```python
from build123d import *

# Parameters (mm, degrees)
F0_W           = 90
F0_H           = 25
F1_DEPTH       = 40
F3_D           = 8.8
F3_CBORE_D     = 14.25
F3_CBORE_DEPTH = 20
F4_T1_DEPTH    = 115.7168298797
F6_D           = 6.8


# Not quite as in the source:
# - a fillet or chamfer that OpenCascade refuses, or shapes differently, is made with other operations: its cross-section is extruded or revolved along the edge and cut away or added


with BuildPart() as f1:
    # F0 (on Front) → F1 (new body)
    with BuildSketch(Plane.XZ):
        with Locations((45, 12.5)):
            Rectangle(F0_W, F0_H)
    extrude(amount=F1_DEPTH)

    # F3 (through all)
    with Locations(Plane.XZ.offset(40)):
        with Locations((22.5, 15), (67.5, 15)):
            CounterBoreHole(F3_D / 2, F3_CBORE_D / 2, F3_CBORE_DEPTH)

    # F4: chamfer of 5 on 1 edges, made by hand

    # F4_s2 → F4_t1 (cut)
    with BuildSketch(Plane.YZ.offset(-12.8584149398)):
        Polygon((-35, 25), (-40, 20), (-40, 25), align=None)
    extrude(amount=F4_T1_DEPTH, mode=Mode.SUBTRACT)

    # F6 (through all)
    with Locations(Plane.XY.offset(25)):
        with Locations((15.8117040992, -15.4151152819), (68.1231990457, -15.4151152819)):
            Hole(F6_D / 2)


solid = f1.part
```
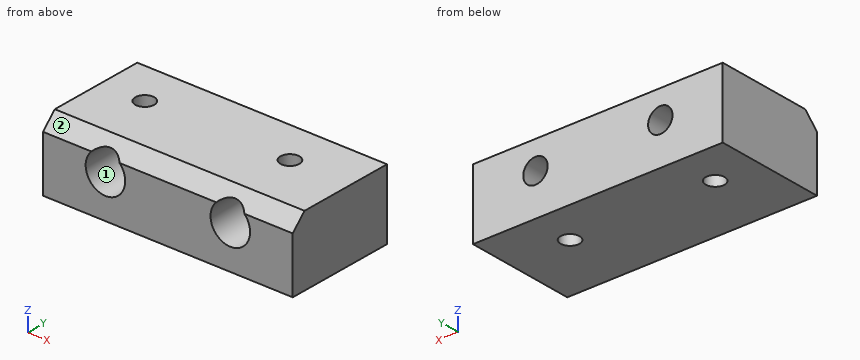
Check sheet for the modelled part. Datum: model origin and axes. Units: mm. Face numbers are marked on the shaded views. A direction names the side the tool comes from. Round coordinates to 2 decimals unless told otherwise and drop trailing zeros. Write each loop counter-clockwise with the first axis right and the second up, starting at its lowest first coordinate (ties: lowest second). Pieces come first, ordered by that corner, then holes. Notation, with made-up numbers: (63, -6.5) -> (113, -6.5) arc R26 cw to (113, 9.5) -> close; hole circle Ø6 at (-3.75, 48.25). An arc over 180 degrees is marked (long way). Put each result on its own line as item: value.
(1) Sectioned sample at C-C (x = 24). Enter the section's corners in (y, z).
Values found:
outline: (-40, 0) -> (0, 0) -> (0, 10.86) -> (-20, 10.86) -> (-20, 8.03) -> (-40, 8.03) -> close; (-38.03, 21.97) -> (-20, 21.97) -> (-20, 19.14) -> (0, 19.14) -> (0, 25) -> (-35, 25) -> close
(2) Material ranges on line 1 (X direction, y = -24.75, z = 15) (3 decimals); line 2 (X direction, y = -16.5, z = 8); line 3 (Y direction, x = 68.5, z = 10.5), recorded low to high.
Values found:
line 1: x = 0 to 15.375, 29.625 to 60.375, 74.625 to 90
line 2: x = 0 to 12.59, 19.03 to 64.9, 71.35 to 90
line 3: y = -20 to -18.79, -12.04 to 0
(3) Tool access check on the marked faces 1 and 2. Record the directions out of +Z, -Z, +X, -X, +Y, -Y that give a thin tool (end or side, any length) a straight path to the whole face; none if there is none.
Values found:
face 1: -Y
face 2: +Z, +X, -X, -Y
(4) Go/stop test with flat-tipped pins: pin 1 Ø6 at (x, y) = (68.12, -15.42) entering from -Z; pin 2 Ø4.5 at (x, z) = (20.5, 14) entering from -Y. Record where each tip stops, or that it passes through.
Values found:
pin 1: passes through
pin 2: stops at y = -20
(5) Sectioned sample at B-B (y = -6.5). Enter the section's corners in (x, z).
Values found:
outline: (0, 0) -> (90, 0) -> (90, 25) -> (0, 25) -> close; hole circle Ø8.8 at (22.5, 15); hole circle Ø8.8 at (67.5, 15)
(6) Sectioned sample at D-D (z = 23.5). Enter the section's corners in (x, y), plus the area to 3 significant figures.
Values found:
outline: (0, -36.5) -> (90, -36.5) -> (90, 0) -> (0, 0) -> close; hole circle Ø6.8 at (15.81, -15.42); hole circle Ø6.8 at (68.12, -15.42)
area: 3,210 mm^2
(7) Sectioned sample at A-A (x = 67.5). Enter the section's corners in (y, z) (3 decimals).
Values found:
outline: (-40, 0) -> (-18.758, 0) -> (-18.758, 10.6) -> (-20, 10.6) -> (-20, 7.875) -> (-40, 7.875) -> close; (-37.875, 22.125) -> (-20, 22.125) -> (-20, 19.4) -> (-18.758, 19.4) -> (-18.758, 25) -> (-35, 25) -> close; (-12.073, 0) -> (0, 0) -> (0, 10.6) -> (-12.073, 10.6) -> close; (-12.073, 19.4) -> (0, 19.4) -> (0, 25) -> (-12.073, 25) -> close
